The listing builds one solid part. Answer for the finished solid, in the listing's coordinates (mm). Round coordinates to 2 decimals unless told otherwise and drop trailing zeros. Write each loop counter-clockwise with the first axis right and the second up, starting at its lowest first coordinate (ties: lowest second). Pieces come first, ordered by that corner, then holes. Notation, with made-up numbers: (14.25, -6.75) - (26.25, -6.75) arc R29 ccw to (26.25, 18.25) - close; hole circle Ø4 at (-4.75, -39). An arc over 180 degrees is marked (long way). Use a Markdown table: item, result. Add a question column.
1) Find the intervals of material crossed by probe 1 along Z at (x, y) = (1.5, 4.25); probe 2 along Y at (x, z) = (-3.5, 2.75), in increasing order. Write a range as from..to.
2) A cutting plane is placed at A-A (x = -2). Give the vertices of the cut face in (y, z).
3) A cutting plane is placed at B-B (z = 2.55). Give the vertices of the cut face in (x, y), then the cut area to 3 significant figures.
```python
from build123d import *

# Parameters (mm, degrees)
SKETCH_1_W      = 22
SKETCH_1_H      = 9
EXTRUDE_1_DEPTH = 3
CHAMFER_1_SIZE  = 1


with BuildPart() as part:
    # Эскиз1 → Вытянуть1 (new body)
    with BuildSketch(Plane.XY):
        Rectangle(SKETCH_1_W, SKETCH_1_H)
    extrude(amount=EXTRUDE_1_DEPTH)

    # Фаска1
    chamfer_1_edges = [part.edges().sort_by_distance(p)[0] for p in [
        (0, 4.5, 3),
        (0, -4.5, 3),
    ]]
    chamfer(chamfer_1_edges, length=CHAMFER_1_SIZE)


solid = part.part
```
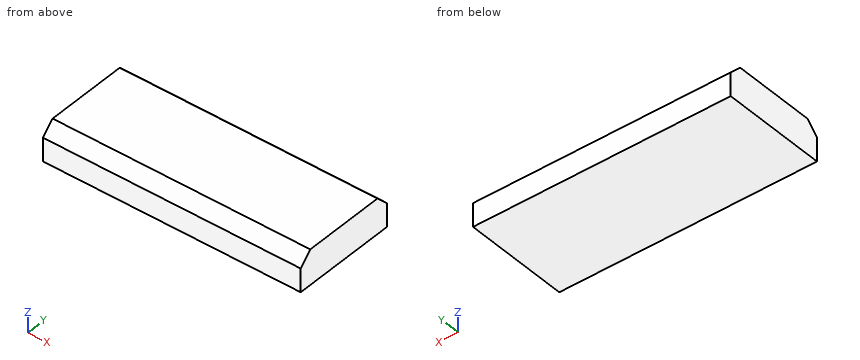
Entries:
| question | item | result |
|---|---|---|
| 1 | probe 1 | z = 0..2.25 |
| 1 | probe 2 | y = -3.75..3.75 |
| 2 | outline | (-4.5, 0) - (4.5, 0) - (4.5, 2) - (3.5, 3) - (-3.5, 3) - (-4.5, 2) - close |
| 3 | outline | (-11, -3.95) - (11, -3.95) - (11, 3.95) - (-11, 3.95) - close |
| 3 | area | 174 mm² |
